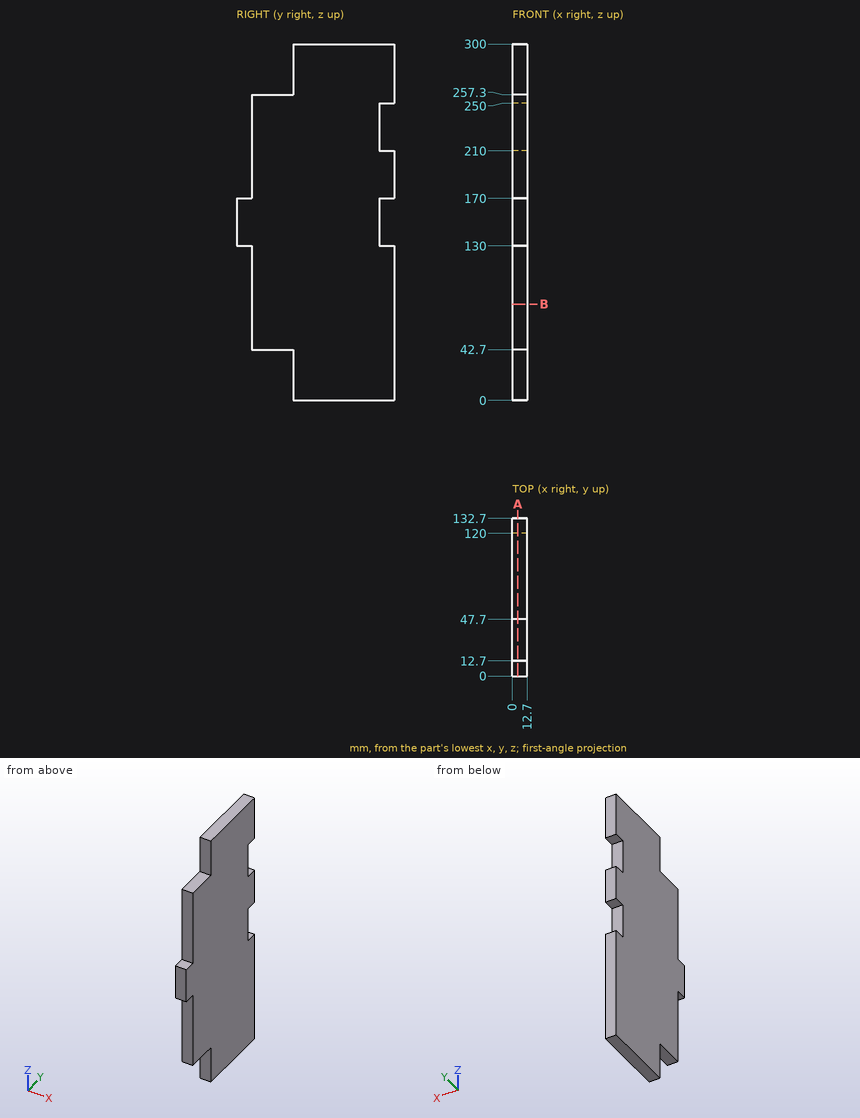
Can you work these out from the drawing? Everything is in mm from the part's minimum corner. Round coordinates to 2 decimals unless told otherwise and drop trailing zeros. Order: outer loops, then holes, each group sorted by start corner. A loop starts at its lowest first (then second) coordinate and runs counter-clockwise, first axis right, second up. Notation, with made-up numbers: M 48,-8.5 L 54,-8.5 A19 ccw 54,13.5 Z; hole C -4.75,80.5 d11. An arc over 180 degrees is marked long. One line per question, with ' | ' between items.
1) For pin 1 Ø1 at (x, z) = (11, 94) entering from -Y; pin 2 Ø4 at (x, z) = (7, 277.5) entering from -Y; pin 3 Ø6.5 at (x, y) = (9.5, 3.5) entering from +Z, each with a flat end and sliding along its axis, tell me the tip position at first contact or that it passes through.
Working result:
pin 1: y = 12.7 | pin 2: y = 47.7 | pin 3: z = 170
2) I need wall thicknesses on line 1 along Z through (x, y) = (9.75, 125.5); line 2 along Y through (x, z) = (7.5, 88.5); line 3 along Z through (x, y) = (8.25, 45.5). Which ranges of each line are inside material? Lowest first, please.
Working result:
line 1: 0 to 130, 170 to 210, 250 to 300 | line 2: 12.7 to 132.7 | line 3: 42.7 to 257.3
3) I want a section at B-B, the plane z = 81. Write out the boundary of the cut face in (x, y), then the cut area to 3 significant figures.
Working result:
outline: M 0,12.7 L 12.7,12.7 L 12.7,132.7 L 0,132.7 Z | area: 1,520 mm²
4) I want a section at A-A, the plane x = 4.75. Write out the boundary of the cut face in (y, z), then the cut area to 3 significant figures.
Working result:
outline: M 0,130 L 12.7,130 L 12.7,42.7 L 47.7,42.7 L 47.7,0 L 132.7,0 L 132.7,130 L 120,130 L 120,170 L 132.7,170 L 132.7,210 L 120,210 L 120,250 L 132.7,250 L 132.7,300 L 47.7,300 L 47.7,257.3 L 12.7,257.3 L 12.7,170 L 0,170 Z | area: 32,500 mm²
